```python
from build123d import *

# Parameters (mm, degrees)
F1_DEPTH = 63.5
F2_DEPTH = 25.4
F3_DEPTH = 7.9375
F5_R     = 6.35


# Not quite as in the source:
# - a feature names something its author has since deleted; it is built from what else it names


with BuildPart() as f1:
    # F0 (on Front) → F1 (new body, symmetric)
    with BuildSketch(Plane.XZ):
        Polygon((24.9004629219, 11.984025088), (-38.5995370781, 11.984025088), (-38.5995370781, -7.065974912), (43.9504629219, -7.065974912), (43.9504629219, 11.984025088), align=None)
    extrude(amount=F1_DEPTH, both=True)

    # F0 (on Front) → F2 (join, symmetric)
    with BuildSketch(Plane.XZ):
        with BuildLine():
            Line((24.9004629219, 29.459225088), (24.9004629219, 11.984025088))
            Line((24.9004629219, 11.984025088), (43.9504629219, 11.984025088))
            Line((43.9504629219, 11.984025088), (43.9504629219, 29.459225088))
            ThreePointArc((43.9504629219, 29.459225088), (48.6001427706, 40.6845452393), (59.8254629219, 45.334225088))
            Line((59.8254629219, 45.334225088), (65.5219778419, 45.334225088))
            Line((65.5219778419, 45.334225088), (88.4004629219, 45.334225088))
            Line((88.4004629219, 45.334225088), (88.4004629219, 64.384225088))
            Line((88.4004629219, 64.384225088), (65.4512095848, 64.384225088))
            Line((65.4512095848, 64.384225088), (59.8254629219, 64.384225088))
            add(Edge.make_bspline(
                [(58.4085351023, 64.3554704527), (58.8803787931, 64.3662992509), (59.3526984445, 64.3758829837), (59.8254629219, 64.384225088)],
                knots=[110.4908750185, 110.4908750185, 110.4908750185, 110.4908750185, 111.5045361635, 111.5045361635, 111.5045361635, 111.5045361635], degree=3))
            ThreePointArc((58.4085351023, 64.3554704527), (34.6337794817, 53.6487829684), (24.9004629219, 29.459225088))
        make_face()
    extrude(amount=F2_DEPTH, both=True)

    # F0 (on Front) → F3 (join, symmetric)
    with BuildSketch(Plane.XZ):
        with BuildLine():
            add(Edge.make_bspline(
                [(-38.5995370781, 11.984025088), (-38.8000023371, 47.2016469024), (6.976730171, 63.1751121082), (58.4085351023, 64.3554704527)],
                knots=[0, 0, 0, 0, 110.4908750185, 110.4908750185, 110.4908750185, 110.4908750185], degree=3))
            Line((-38.5995370781, 11.984025088), (24.9004629219, 11.984025088))
            Line((24.9004629219, 11.984025088), (24.9004629219, 29.459225088))
            ThreePointArc((24.9004629219, 29.459225088), (34.6337794817, 53.6487829684), (58.4085351023, 64.3554704527))
        make_face()
    extrude(amount=F3_DEPTH, both=True)

    # F0 (on Front) → F4 (revolve)
    with BuildSketch(Plane.XZ):
        Polygon((88.4004629219, 69.134025088), (88.4004629219, 64.384225088), (88.4004629219, 45.334225088), (88.4004629219, 40.559025088), (116.2512095848, 40.559025088), (116.2512095848, 69.134025088), align=None)
    revolve(axis=Axis((88.4004629219, 0, 54.846525088), (0, 0, -1)))

    # F5
    f5_edges = [f1.edges().sort_by_distance(p)[0] for p in [
        (-38.599537, -63.5, 2.459025),
        (43.950463, -63.5, 2.459025),
        (-38.599537, 63.5, 2.459025),
        (43.950463, 63.5, 2.459025),
    ]]
    fillet(f5_edges, radius=F5_R)


solid = f1.part
```
For this review, take the finished solid that the model builds, in its own axes (mm). A direction names the side the tool comes from. Round coordinates to 2 decimals unless told otherwise and drop trailing zeros. Order: outer loops, then holes, each group sorted by start corner. A loop starts at its lowest first (then second) coordinate and runs counter-clockwise, first axis right, second up.
Q1. Insertion check: P1, Ø10, axis at x = 60, y = 10.5, coming from the +Z side; P2, Ø1, axis at x = 53, y = 25.5, coming from the -Z side; P3, Ø15.5, axis at x = 58.5, z = 47.5, coming from the -Y side; P4, Ø12, axis at x = 4.5, y = -14.5, coming from the +Z side. Each pin has a flat end and moves straight along its axis. Give the tip position at first contact, or say it passes through.
Findings below:
P1: stops at z = 69.13
P2: stops at z = 43.55
P3: stops at y = -25.4
P4: stops at z = 11.98
Q2. Machinability: for faces 5 (the flat face through (43.95, -1, 7)), 6 (the flat face through (24.9, 17, 21)), 7 (the flat face through (24.9, -17, 21)), 8 (the flat face through (60, 0, 64.384)), which of the approach directions +Z, -Z, +X, -X, +Y, -Y give a long, thin tool a straight path to every point of the face, cutting with its end or side? Answer none if there is none.
Findings below:
face 5: -Z, +X, +Y, -Y
face 6: +Z, -X, +Y
face 7: +Z, -X, -Y
face 8: +Z, -X
Q3. Mouldability with a two-part tool opening along X and no side actions: class faces 1 (the cylindrical face through (42.14, -61.59, 2.59)), 2 (the flat face through (89, 0, 40.559)), 3 (the cylindrical face through (-36.69, -61.69, 2.33)), 4 (the flat face through (60, -4, 45.334)) as pulls with the +X half, pulls with the -X half, needs draft (parallel to the pull), parting line crosses it, or undercut.
Findings below:
face 1: pulls with the +X half
face 2: needs draft
face 3: pulls with the -X half
face 4: undercut
Q4. We need section B-B, the plane y = -37.5. Give the boundary of the cut face in (x, z), plus the area to 3 significant figures.
Findings below:
outline: (-38.6, -7.07) - (43.95, -7.07) - (43.95, 11.98) - (-38.6, 11.98) - close
area: 1,570 mm2
Q5. We need section C-C, the plane x = 81. Give the boundary of the cut face in (y, z).
Findings below:
outline: (-26.85, 40.56) - (26.85, 40.56) - (26.85, 69.13) - (-26.85, 69.13) - close
Q6. Wall thickness on line 1 (X direction, y = 16, z = 9.5); line 2 (Z direction, x = -12.5, y = 45); line 3 (Z direction, x = 67.5, y = 25): over which ranges is each line inside the solid? List them lowest first.
Findings below:
line 1: x = -38.6 to 43.95
line 2: z = -7.07 to 11.98
line 3: z = 45.33 to 64.38
Q7. We need section A-A, the plane z = 5. Give the boundary of the cut face in (x, y), plus the area to 3 significant figures.
Findings below:
outline: (-38.6, -57.15) arc R6.35 ccw to (-32.25, -63.5) - (37.6, -63.5) arc R6.35 ccw to (43.95, -57.15) - (43.95, 57.15) arc R6.35 ccw to (37.6, 63.5) - (-32.25, 63.5) arc R6.35 ccw to (-38.6, 57.15) - close
area: 10,400 mm2
